```python
from build123d import *

# Parameters (mm, degrees)
SKETCH1_W           = 100
SKETCH1_H           = 72
BOSS_EXTRUDE1_DEPTH = 20
SKETCH2_W           = 94
SKETCH2_H           = 66
CUT_EXTRUDE1_DEPTH  = 17
SKETCH3_R           = 2.5
BOSS_EXTRUDE2_DEPTH = 5
SKETCH6_W           = 16
SKETCH6_H           = 8.5
SKETCH6_W_2         = 14
SKETCH6_W_3         = 15
SKETCH6_W_4         = 36
BOSS_EXTRUDE4_DEPTH = 12
SKETCH6_6_W         = 36
SKETCH6_6_H         = 8.5
SKETCH6_6_W_2       = 14
SKETCH6_6_W_3       = 16
SKETCH6_6_W_4       = 15
CUT_EXTRUDE2_DEPTH  = 18
CUT_EXTRUDE4_DEPTH  = 18


with BuildPart() as part:
    # Sketch1 → Boss-Extrude1 (new body)
    with BuildSketch(Plane(origin=(0, 0, 0), x_dir=(1, 0, 0), z_dir=(0, 1, 0))):
        with Locations((0.803212851, 7.285140562)):
            Rectangle(SKETCH1_W, SKETCH1_H)
    extrude(amount=BOSS_EXTRUDE1_DEPTH)

    # Sketch2 → Cut-Extrude1 (cut)
    with BuildSketch(Plane(origin=(0, 20, 0), x_dir=(1, 0, 0), z_dir=(0, 1, 0))):
        with Locations((0.803212851, 7.285140562)):
            Rectangle(SKETCH2_W, SKETCH2_H)
    extrude(amount=-CUT_EXTRUDE1_DEPTH, mode=Mode.SUBTRACT)

    # Sketch3 → Boss-Extrude2 (add)
    with BuildSketch(Plane(origin=(0, 3, 0), x_dir=(1, 0, 0), z_dir=(0, 1, 0))):
        with Locations(Location((-40.962789341, -19.714859438, 0), (0, 0, 270))):
            Circle(SKETCH3_R)
        with Locations(Location((-40.962789341, 19.785140562, 0), (0, 0, 270))):
            Circle(SKETCH3_R)
        with Locations(Location((43.037210659, -17.714859438, 0), (0, 0, 270))):
            Circle(SKETCH3_R)
        with Locations(Location((43.037210659, 19.785140562, 0), (0, 0, 270))):
            Circle(SKETCH3_R)
    extrude(amount=BOSS_EXTRUDE2_DEPTH)

    # Sketch6 → Boss-Extrude4 (add)
    with BuildSketch(Plane(origin=(0, 0, -43.285140562), x_dir=(-1, 0, 0), z_dir=(0, 0, -1))):
        with Locations((-0.803212851, 12.25)):
            Rectangle(SKETCH6_W, SKETCH6_H)
        with Locations((18.196787149, 12.25)):
            Rectangle(SKETCH6_W_2, SKETCH6_H)
        with Locations((36.696787149, 12.25)):
            Rectangle(SKETCH6_W_3, SKETCH6_H)
        with Locations((-28.803212851, 12.25)):
            Rectangle(SKETCH6_W_4, SKETCH6_H)
    extrude(amount=-BOSS_EXTRUDE4_DEPTH)

    # Sketch6_6 → Cut-Extrude2 (cut)
    with BuildSketch(Plane(origin=(0, 0, -43.285140562), x_dir=(-1, 0, 0), z_dir=(0, 0, -1))):
        with Locations((-28.803212851, 12.25)):
            Rectangle(SKETCH6_6_W, SKETCH6_6_H)
        with Locations((18.196787149, 12.25)):
            Rectangle(SKETCH6_6_W_2, SKETCH6_6_H)
        with Locations((-0.803212851, 12.25)):
            Rectangle(SKETCH6_6_W_3, SKETCH6_6_H)
        with Locations((36.696787149, 12.25)):
            Rectangle(SKETCH6_6_W_4, SKETCH6_6_H)
    extrude(amount=-CUT_EXTRUDE2_DEPTH, mode=Mode.SUBTRACT)

    # usb type-c → Cut-Extrude4 (cut)
    with BuildSketch(Plane.XY.offset(28.714859438)):
        with BuildLine():
            Line((-37.196787149, 13), (-17.196787149, 13))
            ThreePointArc((-17.196787149, 13), (-15.782573586, 12.414213562), (-15.196787149, 11))
            Line((-15.196787149, 11), (-15.196787149, 10))
            ThreePointArc((-15.196787149, 10), (-15.782573586, 8.585786438), (-17.196787149, 8))
            Line((-17.196787149, 8), (-37.196787149, 8))
            ThreePointArc((-37.196787149, 8), (-38.611000711, 8.585786438), (-39.196787149, 10))
            Line((-39.196787149, 10), (-39.196787149, 11))
            ThreePointArc((-39.196787149, 11), (-38.611000711, 12.414213562), (-37.196787149, 13))
        make_face()
    extrude(amount=-CUT_EXTRUDE4_DEPTH, mode=Mode.SUBTRACT)


solid = part.part
```
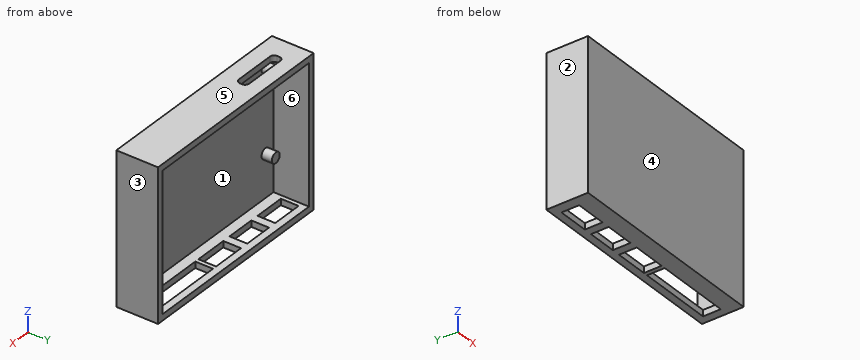
The listing builds one solid part. Answer for the finished solid, in the listing's coordinates (mm). Face numbers are marked on the shaded views. A direction names the side the tool comes from. Give positions to 0.01 mm unless a question says otherwise; leave off trailing zeros. Loops run counter-clockwise (first coordinate to the right, second up) from the corner with the lowest first, then second, coordinate; pieces in that order, holes last. Notation, with made-up numbers: (73.5, 10) - (114.5, 10) arc R8 cw to (114.5, 24) - close; hole circle Ø1 at (-39, -34.5). An arc over 180 degrees is marked (long way). Answer as CSV lines item,"result". Start each with the question number.
Item 1: A cutting plane is placed at D-D on y = 18.75. Determine the outline of the cut face in (x, z), then the cut area to 3 significant figures.
Item 2: A cutting plane is placed at A-A on x = 29.5. Determine the outline of the cut face in (y, z).
Item 3: The mould has two halves that part along X. Classify the marked faces 1, 2, 3 and 4: +X half, -X half, draft (parallel to the pull), parting line (faces both ways), or undercut.
Item 4: Find the intervals of material crossed by line 1 (X direction, y = 3.5, z = -36); line 2 (Z direction, x = -18, y = 7.5); line 3 (Z direction, x = -39.5, y = 3.75), in increasing order. Write a range as from..to.
Item 5: Each of these flat-tipped pins is pushed along its axis until it touches: pin 1 (2.5 mm diameter, centred on x = 42, z = 17, fed in from +Y); pin 2 (1 mm diameter, centred on x = 34, z = -16.5, fed in from +Y). Where does it stop, or does it pass through?
Item 6: A cutting plane is placed at C-C on x = -22.5. Determine the outline of the cut face in (y, z), then the cut area to 4 significant figures.
Item 7: A cutting plane is placed at B-B on y = 14.25. Determine the outline of the cut face in (x, z), then the cut area to 3 significant figures.
Item 8: For the marked faces 5 and 6, determine the directions among +Z, -Z, +X, -X, +Y, -Y from which every point of the face is accessible in a straight line to the end or side of a thin tool.
Found:
1,outline,"(-49.2, -43.29) - (50.8, -43.29) - (50.8, 28.71) - (-49.2, 28.71) - close; hole (-46.2, -40.29) - (47.8, -40.29) - (47.8, 25.71) - (-46.2, 25.71) - close"
1,area,"996 mm^2"
2,outline,"(0, -43.29) - (8, -43.29) - (8, -40.29) - (3, -40.29) - (3, 25.71) - (20, 25.71) - (20, 28.71) - (0, 28.71) - close; (16.5, -43.29) - (20, -43.29) - (20, -40.29) - (16.5, -40.29) - close"
3,face 1,"undercut"
3,face 2,"-X half"
3,face 3,"+X half"
3,face 4,"draft"
4,line 1,"x = -49.2..-46.2, 47.8..50.8"
4,line 2,"z = -43.29..-40.29, 25.71..28.71"
4,line 3,"z = -43.29..-40.29, -21.81..-17.76, 17.69..21.74, 25.71..28.71"
5,pin 1,"stops at y = 8"
5,pin 2,"stops at y = 3"
6,outline,"(0, -43.29) - (8, -43.29) - (8, -40.29) - (3, -40.29) - (3, 25.71) - (8, 25.71) - (8, 28.71) - (0, 28.71) - close; (13, 25.71) - (20, 25.71) - (20, 28.71) - (13, 28.71) - close; (16.5, -43.29) - (20, -43.29) - (20, -40.29) - (16.5, -40.29) - close"
6,area,"277.5 mm^2"
7,outline,"(-49.2, -43.29) - (-44.2, -43.29) - (-44.2, -40.29) - (-46.2, -40.29) - (-46.2, 25.71) - (47.8, 25.71) - (47.8, -40.29) - (46.8, -40.29) - (46.8, -43.29) - (50.8, -43.29) - (50.8, 28.71) - (-49.2, 28.71) - close; (-29.2, -43.29) - (-25.2, -43.29) - (-25.2, -40.29) - (-29.2, -40.29) - close; (-11.2, -43.29) - (-7.2, -43.29) - (-7.2, -40.29) - (-11.2, -40.29) - close; (8.8, -43.29) - (10.8, -43.29) - (10.8, -40.29) - (8.8, -40.29) - close"
7,area,"753 mm^2"
8,face 5,"+Z, +X, -X, +Y, -Y"
8,face 6,"+Y"
